For this review, use the dimensioned drawing (mm, ordinates from the lowest corner) and the shaded views. A direction names the side the tool comes from. Round coordinates to 2 decimals unless told otherwise and drop trailing zeros. Loops run counter-clockwise (first coordinate to the right, second up) from the corner with the lowest first, then second, coordinate; pieces in that order, holes last. Notation, with made-up numbers: M 44,19.5 L 72,19.5 A18 ccw 72,47.5 Z; hole C -34.75,37 d9. An arc over 180 degrees is marked long. Answer as a JSON object with one key per item and string values. Group by question number.
Item 1: Consider section A-A (z = 3.25). Give the boundary of the cut face in (x, y), and give its area (3 significant figures).
Item 2: Insertion check: P1, Ø1, axis at x = 50, y = 15.5, coming from the +Z side; P2, Ø2, axis at x = 12, z = 4.5, coming from the -Y side; P3, Ø3.5, axis at x = 61.5, z = 4.5, coming from the +Y side; P4, Ø1, axis at y = 27, z = 1, coming from the -X side. Each pin has a flat end and moves straight along its axis. Give the tip position at first contact, or say it passes through.
Item 3: Consider section C-C (x = 25.5). Give the boundary of the cut face in (y, z).
Item 4: To check wall thickness, follow line 1 (Y direction, x = 7.5, z = 1.35); line 2 (X direction, y = 52.5, z = 4.3); line 3 (Y direction, x = 57.5, z = 3.1). State the ranges of each line that lie inside material, in increasing order.
Item 5: Tool access review of the marked faces 3, 4 and 5: name each direction out of +Z, -Z, +X, -X, +Y, -Y from which nothing blocks a thin tool from reaching the whole face with its end or side.
Item 6: Consider section B-B (y = 28). Give the boundary of the cut face in (x, z), and give its area (3 significant figures).
Item 7: The part is to be moulded in two halves that separate along Y. For the marked faces 1 and 2, say which applies: +Y half, -Y half, draft (parallel to the pull), parting line (faces both ways), or undercut.
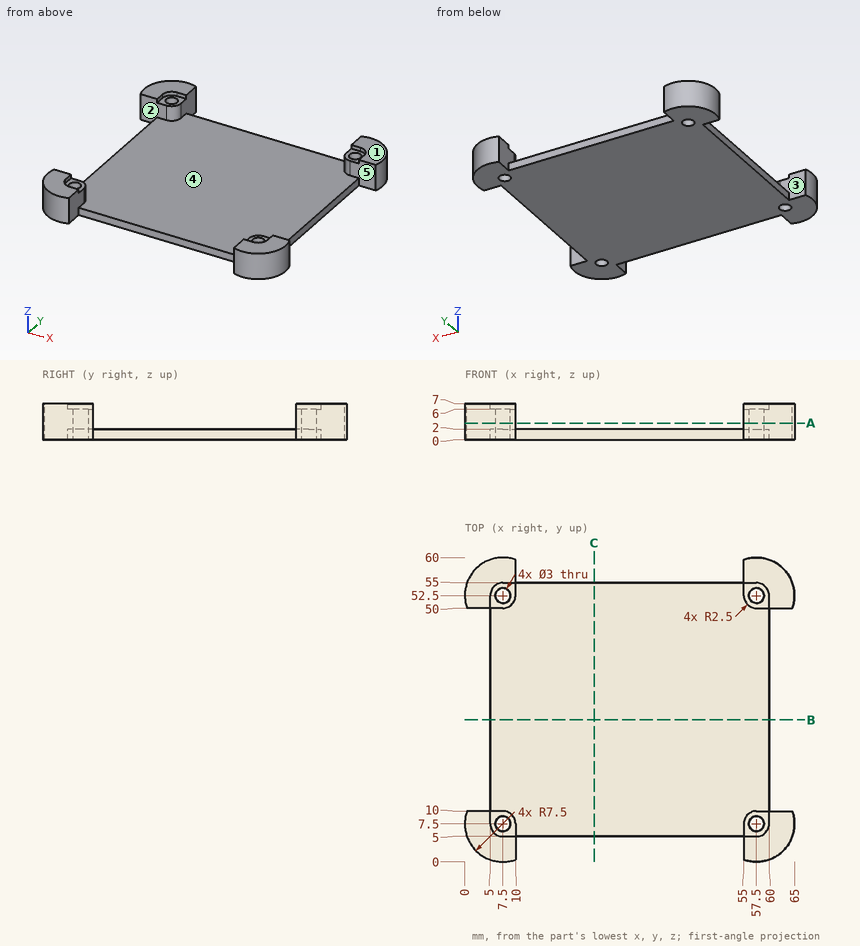
Geometry results:
{
 "1": {"outline": "M 0.43,10 A7.5 ccw 10,0.43 L 10,7.5 A2.5 ccw 7.5,10 Z; M 0.43,50 L 7.5,50 A2.5 ccw 10,52.5 L 10,59.57 A7.5 ccw Z; M 55,0.43 A7.5 ccw 64.57,10 L 57.5,10 A2.5 ccw 55,7.5 Z; M 55,52.5 A2.5 ccw 57.5,50 L 64.57,50 A7.5 ccw 55,59.57 Z; hole C 7.5,7.5 d3; hole C 7.5,52.5 d3; hole C 57.5,7.5 d3; hole C 57.5,52.5 d3", "area": "315 mm^2"},
 "2": {"P1": "stops at z = 2", "P2": "passes through", "P3": "stops at y = 59.65", "P4": "stops at x = 5"},
 "3": {"outline": "M 5,0 L 55,0 L 55,2 L 5,2 Z"},
 "4": {"line 1": "y = 0 to 6, 9 to 51, 54 to 60", "line 2": "x = 0 to 6, 9 to 10, 55 to 56, 59 to 65", "line 3": "y = 0 to 6, 9 to 10, 50 to 51, 54 to 60"},
 "5": {"face 3": "+Z, -X", "face 4": "+Z", "face 5": "+Z, +X"},
 "6": {"outline": "M 5,0 L 60,0 L 60,2 L 5,2 Z", "area": "110 mm^2"},
 "7": {"face 1": "draft", "face 2": "undercut"}
}
